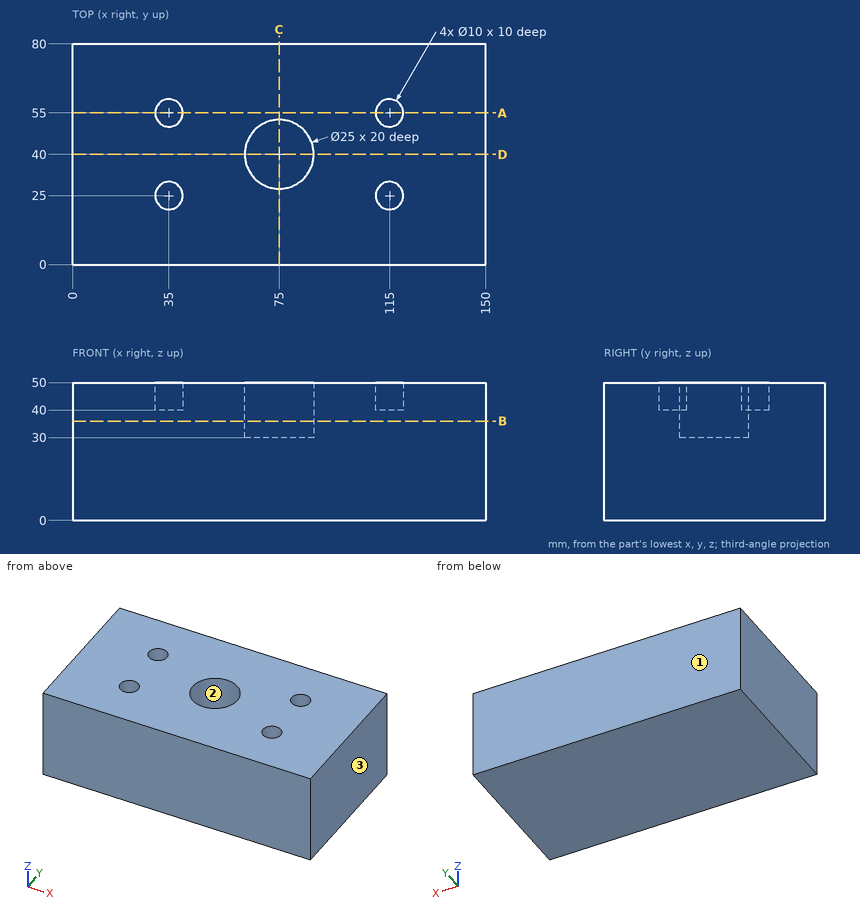
Here's the drawing with two shaded views (mm, measured from the low corner). I have some questions. Round coordinates to 2 decimals unless told otherwise and drop trailing zeros. Loops run counter-clockwise (first coordinate to the right, second up) from the corner with the lowest first, then second, coordinate; pieces in that order, holes last. Notation, with made-up numbers: (37.5, -22) - (65.5, -22) arc R16 cw to (65.5, 1) - close; hole circle Ø6 at (0.25, -29.5). An arc over 180 degrees is marked (long way). Write item = value, one per line.
1) I need wall thicknesses on line 1 along Y through (x, z) = (115, 44.5); line 2 along Z through (x, y) = (66.5, 44.5); line 3 along X through (y, z) = (47, 42). Which ranges of each line are inside material? Lowest first, please. Write a range as from..to.
Computed:
line_1 = 0..20, 30..50, 60..80
line_2 = 0..30
line_3 = 0..64.64, 85.36..150
2) Imagine slicing it at C-C (x = 75). Please give me the cut outline in (y, z), and give its area (3 significant figures).
Computed:
outline = (0, 0) - (80, 0) - (80, 50) - (52.5, 50) - (52.5, 30) - (27.5, 30) - (27.5, 50) - (0, 50) - close
area = 3,500 mm2
3) Imagine slicing it at D-D (y = 40). Please give me the cut outline in (x, z).
Computed:
outline = (0, 0) - (150, 0) - (150, 50) - (87.5, 50) - (87.5, 30) - (62.5, 30) - (62.5, 50) - (0, 50) - close
4) I'm going to push flat-ended pins straight in: P1, Ø5, axis at x = 114.5, y = 26, coming from the +Z side; P2, Ø12.5, axis at x = 71.5, y = 39, coming from the +Z side. Where does each tip first touch, or does it pass through?
Computed:
P1 = 40
P2 = 30
5) Imagine slicing it at B-B (z = 36). Please give me the cut outline in (x, y), and give its area (3 significant figures).
Computed:
outline = (0, 0) - (150, 0) - (150, 80) - (0, 80) - close; hole circle Ø25 at (75, 40)
area = 11,500 mm2
6) Imagine slicing it at A-A (y = 55). Please give me the cut outline in (x, z).
Computed:
outline = (0, 0) - (150, 0) - (150, 50) - (120, 50) - (120, 40) - (110, 40) - (110, 50) - (40, 50) - (40, 40) - (30, 40) - (30, 50) - (0, 50) - close
7) If we mould it in two halves opening along Y, with no side actions, what happens to the marked faces 1, 2 and 3? For each: pulls with the +Y half, pulls with the -Y half, needs draft (parallel to the pull), parting line crosses it, or undercut.
Computed:
face_1 = pulls with the +Y half
face_2 = undercut
face_3 = needs draft
